For this review, take the finished solid that the model builds, in its own axes (mm). Face numbers are marked on the shaded views. Give positions to 0.01 mm unless a question says otherwise; leave off trailing zeros. Loops run counter-clockwise (first coordinate to the right, second up) from the corner with the lowest first, then second, coordinate; pieces in that order, holes last.
```python
from build123d import *

# Parameters (mm, degrees)
F0_W      = 179.780744
F0_H      = 70.839242
F1_DEPTH  = 7
F2_R      = 3.75
F3_DEPTH  = 25
F4_R      = 3.75
F5_DEPTH  = 25
F6_R      = 3.75
F7_DEPTH  = 25
F8_R      = 3.75
F9_DEPTH  = 25
F10_R     = 3.75
F11_DEPTH = 25
F12_R     = 3.75
F13_DEPTH = 25
F14_R     = 3.75
F15_DEPTH = 25


with BuildPart() as f1:
    # F0 (on Front) → F1 (new body)
    with BuildSketch(Plane.XZ):
        with Locations((-1.086671, 22.967793)):
            Rectangle(F0_W, F0_H)
    extrude(amount=F1_DEPTH)

    # F2 (on face) → F3 (join)
    with BuildSketch(Plane.XZ.offset(7)):
        with Locations((-61.695352, 46.280116)):
            Circle(F2_R)
    extrude(amount=F3_DEPTH)

    # F4 (on face) → F5 (join)
    with BuildSketch(Plane.XZ.offset(7)):
        with Locations((-43.921127, 51.411094)):
            Circle(F4_R)
    extrude(amount=F5_DEPTH)

    # F6 (on face) → F7 (join)
    with BuildSketch(Plane.XZ.offset(7)):
        with Locations((-27.999029, 41.509111)):
            Circle(F6_R)
    extrude(amount=F7_DEPTH)

    # F8 (on face) → F9 (join)
    with BuildSketch(Plane.XZ.offset(7)):
        with Locations((-6.212159, 38.454227)):
            Circle(F8_R)
    extrude(amount=F9_DEPTH)

    # F10 (on face) → F11 (join)
    with BuildSketch(Plane.XZ.offset(7)):
        with Locations((17.710951, 36.534646)):
            Circle(F10_R)
    extrude(amount=F11_DEPTH)

    # F12 (on face) → F13 (join)
    with BuildSketch(Plane.XZ.offset(7)):
        with Locations((38.921294, 21.497313)):
            Circle(F12_R)
    extrude(amount=F13_DEPTH)

    # F14 (on face) → F15 (join)
    with BuildSketch(Plane.XZ.offset(7)):
        with Locations((66.4901, 16.602323)):
            Circle(F14_R)
    extrude(amount=F15_DEPTH)


solid = f1.part
```
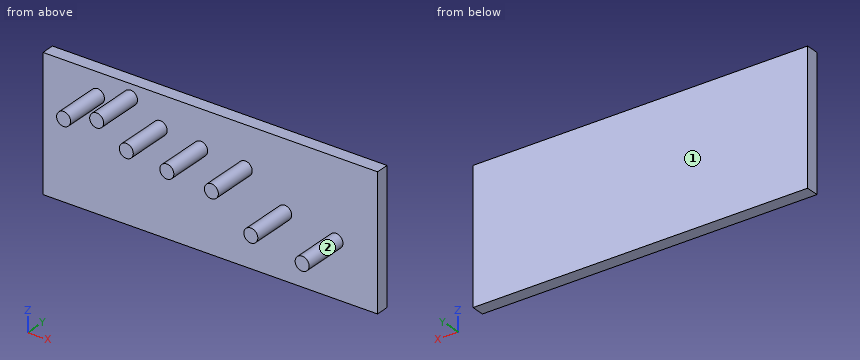
Q1. Mouldability with a two-part tool opening along X and no side actions: class the marked faces 1 and 2 as +X half, -X half, draft (parallel to the pull), parting line (faces both ways), or undercut.
Answers:
face 1: draft
face 2: undercut
Q2. Consider section A-A on y = -18. Give the boundary of the cut face in (x, z), plus the area to 3 significant figures.
Answers:
outline: circle Ø7.5 at (-61.7, 46.28); circle Ø7.5 at (-43.92, 51.41); circle Ø7.5 at (-28, 41.51); circle Ø7.5 at (-6.21, 38.45); circle Ø7.5 at (17.71, 36.53); circle Ø7.5 at (38.92, 21.5); circle Ø7.5 at (66.49, 16.6)
area: 309 mm2
Q3. For probe 1 along Y at (x, z) = (1, -2); probe 2 along Z at (x, y) = (-59.5, -31); probe 3 along Z at (x, y) = (-42, -27), list the stretches that pass through material, from the lowest coordinate up.
Answers:
probe 1: y = -7 to 0
probe 2: z = 43.24 to 49.32
probe 3: z = 48.19 to 54.63
Q4. Consider section C-C on z = -8. Give the boundary of the cut face in (x, y).
Answers:
outline: (-90.98, -7) - (88.8, -7) - (88.8, 0) - (-90.98, 0) - close
Q5. For pin 1 Ø2 at (y, z) = (-25, 51.5) entering from +X; pin 2 Ø5 at (y, z) = (-24.5, 44.5) entering from -X; pin 3 Ø4 at (x, z) = (-24, 48) entering from -Y, all flat-tipped, find the tip position at first contact; note any pin that passes through.
Answers:
pin 1: stops at x = -40.17
pin 2: stops at x = -65.45
pin 3: stops at y = -7
Q6. Consider section B-B on x = -60. Give the boundary of the cut face in (y, z) (3 decimals), plus the area to 3 significant figures.
Answers:
outline: (-32, 42.935) - (-7, 42.935) - (-7, -12.452) - (0, -12.452) - (0, 58.387) - (-7, 58.387) - (-7, 49.625) - (-32, 49.625) - close
area: 663 mm2
